The listing builds one solid part. Answer for the finished solid, in the listing's coordinates (mm). A direction names the side the tool comes from. Give positions to 0.01 mm unless a question says otherwise; leave off trailing zeros. Write each loop counter-clockwise with the first axis right and the second up, starting at its lowest first coordinate (ties: lowest second). Pieces come first, ordered by that corner, then holes. Notation, with made-up numbers: (68, 72.25) - (127, 72.25) arc R21 cw to (127, 104.25) - close; hole circle Ø8 at (20.5, 1). An arc over 180 degrees is marked (long way). Return JSON: item names as keys, results as strings.
from build123d import *

# Parameters (mm, degrees)
SKETCH1_W               = 50
SKETCH1_H               = 53.3
BOSS_EXTRUDE1_DEPTH     = 3.175
SKETCH2_W               = 50
SKETCH2_H               = 3
BOSS_EXTRUDE2_DEPTH     = 48.97
SKETCH3_W               = 3.175
SKETCH3_H               = 15
SKETCH3_H_2             = 15.175
BOSS_EXTRUDE3_DEPTH     = 20
CUT_EXTRUDE1_DEPTH      = 65
SKETCH5_R               = 11
SKETCH5_R_2             = 1.7
CUT_EXTRUDE2_DEPTH      = 65
CUT_EXTRUDE3_DEPTH      = 65
CHAMFER1_SIZE           = 5
FILLET1_R               = 5
BOSS_EXTRU_1_DEPTH      = 6.81
ENL_V_MAT_EXTRU_1_DEPTH = 6.81
BOSS_EXTRU_2_DEPTH      = 3.18
BOSS_EXTRU_3_DEPTH      = 3.18
ESQUISSE5_W             = 13.5
ESQUISSE5_H             = 48.3
BOSS_EXTRU_4_DEPTH      = 6.81
ESQUISSE6_W             = 20
ESQUISSE6_H             = 48.3
ESQUISSE6_R             = 2.5
BOSS_EXTRU_5_DEPTH      = 6.81
ESQUISSE7_W             = 3.5
ESQUISSE7_H             = 48.3
BOSS_EXTRU_6_DEPTH      = 20
ESQUISSE8_R             = 2.5
ENL_V_MAT_EXTRU_2_DEPTH = 10
ESQUISSE9_R             = 4.5
ESQUISSE9_R_2           = 4.595775112
ENL_V_MAT_EXTRU_3_DEPTH = 3.31
CONG_1_R                = 6
CONG_2_R                = 13
BOSS_EXTRU_7_DEPTH      = 3
BOSS_EXTRU_7_DEPTH_BACK = 3


with BuildPart() as part:
    # Sketch1 → Boss-Extrude1 (new body)
    with BuildSketch(Plane(origin=(0, 0, 0), x_dir=(1, 0, 0), z_dir=(0, 1, 0))):
        with Locations((25, 26.65)):
            Rectangle(SKETCH1_W, SKETCH1_H)
    extrude(amount=BOSS_EXTRUDE1_DEPTH)

    # Sketch2 → Boss-Extrude2 (add)
    with BuildSketch(Plane(origin=(0, 3.175, 0), x_dir=(1, 0, 0), z_dir=(0, 1, 0))):
        with Locations((25, 1.5)):
            Rectangle(SKETCH2_W, SKETCH2_H)
    extrude(amount=BOSS_EXTRUDE2_DEPTH)

    # Sketch3 → Boss-Extrude3 (add)
    with BuildSketch(Plane(origin=(0, 3.175, 0), x_dir=(1, 0, 0), z_dir=(0, 1, 0))):
        with Locations((1.5875, 10.5)):
            Rectangle(SKETCH3_W, SKETCH3_H)
        with Locations((48.4125, 10.5875)):
            Rectangle(SKETCH3_W, SKETCH3_H_2)
    extrude(amount=BOSS_EXTRUDE3_DEPTH)

    # Sketch4 → Cut-Extrude1 (cut)
    with BuildSketch(Plane(origin=(50, 0, 0), x_dir=(0, 0, -1), z_dir=(1, 0, 0))):
        Polygon((18.175, 3.175), (3, 23.175), (18.175, 23.175), align=None)
    extrude(amount=-CUT_EXTRUDE1_DEPTH, mode=Mode.SUBTRACT)

    # Sketch5 → Cut-Extrude2 (cut)
    with BuildSketch(Plane.XY):
        with Locations((25, 31.145)):
            Circle(SKETCH5_R)
        with Locations((40.502, 46.647)):
            Circle(SKETCH5_R_2)
        with Locations((9.528, 46.677)):
            Circle(SKETCH5_R_2)
        with Locations((9.498, 15.703)):
            Circle(SKETCH5_R_2)
        with Locations((40.472, 15.673)):
            Circle(SKETCH5_R_2)
    extrude(amount=-CUT_EXTRUDE2_DEPTH, mode=Mode.SUBTRACT)

    # Sketch6 → Cut-Extrude3 (cut)
    with BuildSketch(Plane(origin=(0, 3.175, 0), x_dir=(1, 0, 0), z_dir=(0, 1, 0))):
        with BuildLine():
            ThreePointArc((42.125, 42.3), (40, 44.425), (37.875, 42.3))
            Line((37.875, 42.3), (37.875, 12.3))
            ThreePointArc((37.875, 12.3), (40, 10.175), (42.125, 12.3))
            Line((42.125, 12.3), (42.125, 42.3))
        make_face()
        with BuildLine():
            Line((7.875, 42.3), (7.875, 12.3))
            ThreePointArc((7.875, 12.3), (10, 10.175), (12.125, 12.3))
            Line((12.125, 12.3), (12.125, 42.3))
            ThreePointArc((12.125, 42.3), (10, 44.425), (7.875, 42.3))
        make_face()
    extrude(amount=-CUT_EXTRUDE3_DEPTH, mode=Mode.SUBTRACT)

    # Chamfer1
    chamfer1_edges = [part.edges().sort_by_distance(p)[0] for p in [
        (0, 1.5875, -53.3),
        (50, 1.5875, -53.3),
        (0, 52.145, -1.5),
        (50, 52.145, -1.5),
    ]]
    chamfer(chamfer1_edges, length=CHAMFER1_SIZE)

    # Fillet1
    fillet1_edges = [part.edges().sort_by_distance(p)[0] for p in [
        (25, 3.175, -3),
        (25, 0, 0),
    ]]
    fillet(fillet1_edges, radius=FILLET1_R)

    # Esquisse2 → Boss.-Extru.1 (add)
    with BuildSketch(Plane(origin=(0, 3.175, 0), x_dir=(1, 0, 0), z_dir=(0, 1, 0))):
        Polygon((0, 48.3), (5, 53.3), (45, 53.3), (50, 48.3), (50, 0), (0, 0), align=None)
    extrude(amount=BOSS_EXTRU_1_DEPTH)

    # Esquisse2<2> → Enlèv. mat.-Extru.1 (cut)
    with BuildSketch(Plane(origin=(0, 3.175, 0), x_dir=(1, 0, 0), z_dir=(0, 1, 0))):
        Polygon((0, 48.3), (5, 53.3), (45, 53.3), (50, 48.3), (50, 0), (0, 0), align=None)
    extrude(amount=-ENL_V_MAT_EXTRU_1_DEPTH, mode=Mode.SUBTRACT)

    # Esquisse3 → Boss.-Extru.2 (add)
    with BuildSketch(Plane.ZY):
        Polygon((-20, 9.985), (-3, 26.985), (-3, 9.985), align=None)
    extrude(amount=-BOSS_EXTRU_2_DEPTH)

    # Esquisse4 → Boss.-Extru.3 (add)
    with BuildSketch(Plane.ZY.offset(-46.825)):
        Polygon((-20, 9.985), (-2.507234201, 9.985), (-3, 26.985), align=None)
    extrude(amount=-BOSS_EXTRU_3_DEPTH)

    # Esquisse5 → Boss.-Extru.4 (add)
    with BuildSketch(Plane(origin=(0, 9.985, 0), x_dir=(1, 0, 0), z_dir=(0, 1, 0))):
        with Locations((56.75, 24.15)):
            Rectangle(ESQUISSE5_W, ESQUISSE5_H)
    extrude(amount=-BOSS_EXTRU_4_DEPTH)

    # Esquisse6 → Boss.-Extru.5 (add)
    with BuildSketch(Plane(origin=(0, 9.985, 0), x_dir=(1, 0, 0), z_dir=(0, 1, 0))):
        with Locations((73.5, 24.15)):
            Rectangle(ESQUISSE6_W, ESQUISSE6_H)
        with Locations(Location((73.5, 39.3, 0), (0, 0, 270))):
            Circle(ESQUISSE6_R, mode=Mode.SUBTRACT)
        with Locations(Location((73.5, 9, 0), (0, 0, 270))):
            Circle(ESQUISSE6_R, mode=Mode.SUBTRACT)
    extrude(amount=-BOSS_EXTRU_5_DEPTH)

    # Esquisse7 → Boss.-Extru.6 (add)
    with BuildSketch(Plane(origin=(0, 3.175, 0), x_dir=(-1, 0, 0), z_dir=(0, -1, 0))):
        with Locations((-61.75, 24.15)):
            Rectangle(ESQUISSE7_W, ESQUISSE7_H)
    extrude(amount=BOSS_EXTRU_6_DEPTH)

    # Esquisse8 → Enlèv. mat.-Extru.2 (cut)
    with BuildSketch(Plane(origin=(63.5, 0, 0), x_dir=(0, 0, -1), z_dir=(1, 0, 0))):
        with Locations((9, -6.825)):
            Circle(ESQUISSE8_R)
        with Locations((39.3, -6.825)):
            Circle(ESQUISSE8_R)
    extrude(amount=-ENL_V_MAT_EXTRU_2_DEPTH, mode=Mode.SUBTRACT)

    # Esquisse9 → Enlèv. mat.-Extru.3 (cut)
    with BuildSketch(Plane(origin=(0, 9.985, 0), x_dir=(1, 0, 0), z_dir=(0, 1, 0))):
        with Locations(Location((73.5, 39.3, 0), (0, 0, 270))):
            Circle(ESQUISSE9_R)
        with Locations(Location((73.5, 9, 0), (0, 0, 270))):
            Circle(ESQUISSE9_R_2)
    extrude(amount=-ENL_V_MAT_EXTRU_3_DEPTH, mode=Mode.SUBTRACT)

    # Congé1
    cong_1_edges = [part.edges().sort_by_distance(p)[0] for p in [
        (60, 3.175, -24.15),
    ]]
    fillet(cong_1_edges, radius=CONG_1_R)

    # Congé2
    # the kernel refuses this fillet: 13 mm, written as the material it adds along each edge
    with BuildSketch(Plane(origin=(50, 9.985, 0), x_dir=(1, 0, 0), z_dir=(0, 0, -1))) as cong_2_piece_1_section:
        with BuildLine():
            CenterArc((CONG_2_R, -CONG_2_R), CONG_2_R, 90, 90)
            Line((0, -CONG_2_R), (0, 0))
            Line((0, 0), (CONG_2_R, 0))
        make_face()
    cong_2_piece_1 = extrude(amount=35.007234201, mode=Mode.PRIVATE)
    cong_2_piece_1 = split(cong_2_piece_1, bisect_by=Plane(origin=(52.869924632, 20.818582146, -9.166417854), z_dir=(0, -0.7071067811865461, 0.707106781186549)), keep=Keep.TOP, mode=Mode.PRIVATE)
    add(cong_2_piece_1)

    # Esquisse11 → Boss.-Extru.7 (add, two sides: drawn at the far end of the back side and taken through both)
    with BuildSketch(Plane(origin=(0, 0, -24.15), x_dir=(-1, 0, 0), z_dir=(0, 0, -1)).offset(-BOSS_EXTRU_7_DEPTH_BACK)):
        Polygon((-63.5, -16.825), (0, 9.985), (-63.5, 9.985), align=None)
    extrude(amount=BOSS_EXTRU_7_DEPTH + BOSS_EXTRU_7_DEPTH_BACK)


solid = part.part
Item 1: Flat-ended cylindrical pins translate along their axes: P1, Ø5, axis at y = 24.5, z = -4, coming from the +X side; P2, Ø5.5, axis at x = 27.5, y = -6, coming from the -Z side; P3, Ø8, axis at x = 15.5, z = -28.5, coming from the +Y side (3 decimals); P4, Ø6.5, axis at x = 73.5, z = -9, coming from the -Y side (3 decimals). Find the tip coordinate at first contact, or state that the pin passes through.
Answer below:
{"P1": "stops at x = 50.04", "P2": "passes through", "P3": "stops at y = 9.985", "P4": "stops at y = 3.175"}
Item 2: A cutting plane is placed at B-B on z = -39.3. Determine the outline of the cut face in (x, y) (3 decimals), then the cut area to 3 significant figures.
Answer below:
{"outline": "(0, 3.175) - (54, 3.175) arc R6 cw to (60, -2.825) - (60, -4.325) - (63.5, -4.325) - (63.5, 3.175) - (71, 3.175) - (71, 6.675) - (69, 6.675) - (69, 9.985) - (0, 9.985) - close; (60, -16.825) - (63.5, -16.825) - (63.5, -9.325) - (60, -9.325) - close; (76, 3.175) - (83.5, 3.175) - (83.5, 9.985) - (78, 9.985) - (78, 6.675) - (76, 6.675) - close", "area": "582 mm²"}
Item 3: A cutting plane is placed at D-D on z = -33. Determine the outline of the cut face in (x, y) (3 decimals).
Answer below:
{"outline": "(0, 3.175) - (54, 3.175) arc R6 cw to (60, -2.825) - (60, -16.825) - (63.5, -16.825) - (63.5, 3.175) - (83.5, 3.175) - (83.5, 9.985) - (0, 9.985) - close"}
Item 4: A cutting plane is placed at A-A on x = 73.5. Determine the outline of the cut face in (y, z) (3 decimals).
Answer below:
{"outline": "(3.175, -48.3) - (9.985, -48.3) - (9.985, -43.8) - (6.675, -43.8) - (6.675, -41.8) - (3.175, -41.8) - close; (3.175, -36.8) - (6.675, -36.8) - (6.675, -34.8) - (9.985, -34.8) - (9.985, -13.596) - (6.675, -13.596) - (6.675, -11.5) - (3.175, -11.5) - close; (3.175, -6.5) - (6.675, -6.5) - (6.675, -4.404) - (9.985, -4.404) - (9.985, 0) - (3.175, 0) - close"}
Item 5: The mould has two halves that part along X. Classify faces 5 (the face through (61.774, -6.074, -41.685)), 6 (the face through (77.96, 8.35, -39.89)), 7 (the face through (72, 6.675, -37)), 8 (the face through (38.372, -6.216, -24.108)): +X half, -X half, draft (parallel to the pull), parting line (faces both ways), or undercut.
Answer below:
{"face 5": "draft", "face 6": "undercut", "face 7": "undercut", "face 8": "-X half"}
Item 6: Consider L1, parallel to Y at x = 25, z = -1 (3 decimals); L2, parallel to X at y = 7.3, z = -39.3; L3, parallel to X at y = 8.95, z = -9. Determine where each line is inside the solid, lowest interval first.
Answer below:
{"L1": "y = 3.175 to 20.145, 42.145 to 52.145", "L2": "x = 0 to 69, 78 to 83.5", "L3": "x = 0 to 68.9, 78.1 to 83.5"}
Item 7: A cutting plane is placed at C-C on x = 25. Determine the outline of the cut face in (y, z) (3 decimals).
Answer below:
{"outline": "(-0.57, -27.15) - (3.175, -27.15) - (3.175, -53.3) - (9.985, -53.3) - (9.985, -3) - (20.145, -3) - (20.145, 0) - (3.175, 0) - (3.175, -21.15) - (-0.57, -21.15) - close; (42.145, -3) - (52.145, -3) - (52.145, 0) - (42.145, 0) - close"}
Item 8: For faces 1 (the face through (43, -4, -27.15)), 2 (the face through (58.2, 1.46, -10.72)), 3 (the face through (71.5, 6.675, -7)), 4 (the face through (60, -10, -18)), determine the directions among +Z, -Z, +X, -X, +Y, -Y from which every point of the face is accessible in a straight line to the end or side of a thin tool.
Answer below:
{"face 1": "-Z, -X, -Y", "face 2": "+Z, -X, -Y", "face 3": "+Y", "face 4": "-X, -Y"}
